from build123d import *

# Parameters (mm, degrees)
FILLET1_R = 0.508
FILLET2_R = 2.54
FILLET3_R = 12.7
FILLET4_R = 0.508
FILLET5_R = 0.762


with BuildPart() as part:
    # Sketch1 → Revolve1 (revolve)
    with BuildSketch(Plane.XY, mode=Mode.PRIVATE) as revolve1_sk:
        Polygon((0, 0), (0.508, 0), (2.286, 2.54), (2.286, 3.81), (3.2131, 3.81), (3.2131, 9.398), (4.193012455, 14.859), (5.08, 40.259), (5.588, 40.259), (4.191, 129.54), (0, 129.54), align=None)
    revolve(revolve1_sk.sketch.rotate(Axis((0, 0, 0), (0, 1, 0)), 90), axis=Axis((0, 0, 0), (0, 1, 0)))

    # Fillet1
    fillet1_edges = [part.edges().sort_by_distance(p)[0] for p in [
        (0, 0, 0.508),
    ]]
    fillet(fillet1_edges, radius=FILLET1_R)

    # Fillet2
    fillet2_edges = [part.edges().sort_by_distance(p)[0] for p in [
        (0, 2.54, 2.286),
    ]]
    fillet(fillet2_edges, radius=FILLET2_R)

    # Fillet3
    fillet3_edges = [part.edges().sort_by_distance(p)[0] for p in [
        (0, 14.859, 4.193012455),
        (0, 9.398, 3.2131),
    ]]
    fillet(fillet3_edges, radius=FILLET3_R)

    # Fillet4
    fillet4_edges = [part.edges().sort_by_distance(p)[0] for p in [
        (0, 3.81, 3.2131),
    ]]
    fillet(fillet4_edges, radius=FILLET4_R)

    # Fillet5
    fillet5_edges = [part.edges().sort_by_distance(p)[0] for p in [
        (0, 129.54, 4.191),
    ]]
    fillet(fillet5_edges, radius=FILLET5_R)


solid = part.part
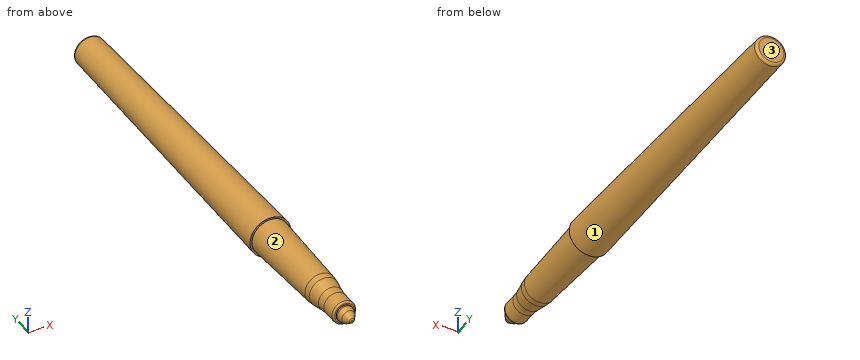
Part model, mm, in its own coordinate system. Face numbers are marked on the shaded views. A direction names the side the tool comes from. Coordinates: 2 decimals unless noted, no trailing zeros. Order: outer loops, then holes, each group sorted by start corner. A loop starts at its lowest first (then second) coordinate and runs counter-clockwise, first axis right, second up.
(1) Tool access for the marked faces 1, 2 and 3: list every direction of +Z, -Z, +X, -X, +Y, -Y with a clear straight run to the whole face (end or side of a thin tool).
Check sheet entries:
face 1: +Y
face 2: -Y
face 3: +Z, -Z, +X, -X, +Y
(2) Slice it at A-A, the plane y = 95.5. Write the cut outline in (x, z).
Check sheet entries:
outline: circle Ø9.45 at (0, 0)
(3) Slice it at B-B, the plane y = 75.5. Write the cut outline in (x, z).
Check sheet entries:
outline: circle Ø10.07 at (0, 0)
(4) Probe L1, parallel to Y at x = 0.25, z = 2.75; L2, parallel to X at y = 106, z = -1.75; L3, parallel to X at y = 77, z = -3. List the from-to ranges inside material, lowest first.
Check sheet entries:
L1: y = 3.81 to 129.54
L2: x = -4.21 to 4.21
L3: x = -4.02 to 4.02
(5) Pin check, flat tips, straight feed: pin 1 Ø1.6 at (x, z) = (1, -1) entering from -Y; pin 2 Ø6 at (x, y) = (-3, 67) entering from -Z; pin 3 Ø5 at (y, z) = (97, -4.5) entering from +X. Stop position of each tip, or through.
Check sheet entries:
pin 1: stops at y = 0.16
pin 2: stops at z = -5.18
pin 3: stops at x = 4.25
